```python
from build123d import *

# Parameters (mm, degrees)
SKETCH_W      = 35
SKETCH_H      = 80
SKETCH_R      = 2
PAD_DEPTH     = 3
SKETCH001_R   = 14
SKETCH001_R_2 = 2
PAD001_DEPTH  = 3


with BuildPart() as part:
    # Sketch → Pad (new body)
    with BuildSketch(Plane.XY):
        Rectangle(SKETCH_W, SKETCH_H)
        with Locations((0, 30)):
            Circle(SKETCH_R, mode=Mode.SUBTRACT)
        with Locations((0, -30)):
            Circle(SKETCH_R, mode=Mode.SUBTRACT)
        with Locations((8, 30)):
            Circle(SKETCH_R, mode=Mode.SUBTRACT)
        with Locations((8, -30)):
            Circle(SKETCH_R, mode=Mode.SUBTRACT)
    extrude(amount=-PAD_DEPTH)

    # Sketch001 (on Face4 of Pad) → Pad001 (join)
    with BuildSketch(Plane(origin=(-17.5, 0, 0), x_dir=(0, -1, 0), z_dir=(-1, 0, 0))):
        with BuildLine():
            Line((40, 0), (-40, 0))
            Line((-40, 0), (-18.024946, 34.613538))
            ThreePointArc((18.024946, 34.613538), (0, 44), (-18.024946, 34.613538))
            Line((40, 0), (18.024946, 34.613538))
        make_face()
        with Locations((0, 22)):
            Circle(SKETCH001_R, mode=Mode.SUBTRACT)
        with Locations((0, 4.5)):
            Circle(SKETCH001_R_2, mode=Mode.SUBTRACT)
        with Locations((0, 39.5)):
            Circle(SKETCH001_R_2, mode=Mode.SUBTRACT)
        with Locations((-17.5, 22)):
            Circle(SKETCH001_R_2, mode=Mode.SUBTRACT)
        with Locations((17.5, 22)):
            Circle(SKETCH001_R_2, mode=Mode.SUBTRACT)
    extrude(amount=-PAD001_DEPTH)


solid = part.part
```
Can you work these out from the model? Positions are in its coordinate system, mm. A direction names the side the tool comes from. Coordinates: 2 decimals unless noted, no trailing zeros. Loops run counter-clockwise (first coordinate to the right, second up) from the corner with the lowest first, then second, coordinate; pieces in that order, holes last.
Item 1: Please list where these lines run through material, in increasing order: L1, parallel to Y at x = 0, z = -2.3; L2, parallel to Z at x = -16, y = 0; L3, parallel to X at y = -13.5, z = 7.
Answers below:
L1: y = -40 to -32, -28 to 28, 32 to 40
L2: z = -3 to 2.5, 6.5 to 8, 36 to 37.5, 41.5 to 44
L3: x = -17.5 to -14.5
Item 2: If we mould it in two halves opening along Z, with no side actions, what happens to faces 1 (the face through (-16.02, 3.03, 8.33)), 2 (the face through (-16.02, 29.17, 17.06)), 3 (the face through (0, -40, -1))? For each: released by +Z, released by -Z, zero draft, split by the parting line, or undercut.
Answers below:
face 1: undercut
face 2: released by +Z
face 3: zero draft
Item 3: Suppose I cut it at C-C (z = 28). Please give me the cut outline in (x, y), then the cut area to 3 significant figures.
Answers below:
outline: (-17.5, -22.22) - (-14.5, -22.22) - (-14.5, -12.65) - (-17.5, -12.65) - close; (-17.5, 12.65) - (-14.5, 12.65) - (-14.5, 22.22) - (-17.5, 22.22) - close
area: 57.4 mm2
Item 4: I'm going to push flat-ended pins straight in: pin 1 (6.5 mm diameter, centred on x = 0, y = 30, fed in from +Z); pin 2 (13 mm diameter, centred on y = 6, z = 15, fed in from +X). Where does each tip first touch, or does it pass through?
Answers below:
pin 1: stops at z = 0
pin 2: stops at x = -14.5
Item 5: Suppose I cut it at B-B (x = 0). Please give me the cut outline in (y, z), then the cut area to 3 significant figures.
Answers below:
outline: (-40, -3) - (-32, -3) - (-32, 0) - (-40, 0) - close; (-28, -3) - (28, -3) - (28, 0) - (-28, 0) - close; (32, -3) - (40, -3) - (40, 0) - (32, 0) - close
area: 216 mm2
Item 6: Suppose I cut it at D-D (y = -31). Please give me the cut outline in (x, z).
Answers below:
outline: (-17.5, -3) - (-1.73, -3) - (-1.73, 0) - (-14.5, 0) - (-14.5, 14.18) - (-17.5, 14.18) - close; (1.73, -3) - (6.27, -3) - (6.27, 0) - (1.73, 0) - close; (9.73, -3) - (17.5, -3) - (17.5, 0) - (9.73, 0) - close
Item 7: Which directions (+Z, -Z, +X, -X, +Y, -Y) give clear straight access to the entire face, cutting with the end or side of a thin tool? Please do faces 4 (the face through (-14.5, -0.6, 7.6)), 5 (the face through (-16, -15.9, 20.8)).
Answers below:
face 4: +Z, +X, +Y, -Y
face 5: +X, -X
Item 8: Suppose I cut it at A-A (y = 0). Please give me the cut outline in (x, z).
Answers below:
outline: (-17.5, -3) - (17.5, -3) - (17.5, 0) - (-14.5, 0) - (-14.5, 2.5) - (-17.5, 2.5) - close; (-17.5, 6.5) - (-14.5, 6.5) - (-14.5, 8) - (-17.5, 8) - close; (-17.5, 36) - (-14.5, 36) - (-14.5, 37.5) - (-17.5, 37.5) - close; (-17.5, 41.5) - (-14.5, 41.5) - (-14.5, 44) - (-17.5, 44) - close
